```python
from build123d import *

# Parameters (mm, degrees)
BOSS_EXTRUDE1_DEPTH    = 3.81
F_10_CLEARANCE_HOLE1_D = 5.1054
F_6_32_TAPPED_HOLE1_D  = 2.7051
SKETCH4_R              = 3.175
CUT_EXTRUDE1_DEPTH     = 33.948179104


with BuildPart() as part:
    # Sketch1 → Boss-Extrude1 (new body)
    with BuildSketch(Plane(origin=(0, 0, 0), x_dir=(0, 0, -1), z_dir=(1, 0, 0))):
        with BuildLine():
            ThreePointArc((-25.906015625, 4.73554162), (-30.1625, 0), (-25.906015625, -4.73554162))
            ThreePointArc((-25.906015625, -4.73554162), (-15.759385528, -6.884569442), (-6.260703125, -11.049597114))
            ThreePointArc((-6.260703125, -11.049597114), (0, -12.7), (6.260703125, -11.049597114))
            ThreePointArc((6.260703125, -11.049597114), (15.759385528, -6.884569442), (25.906015625, -4.73554162))
            ThreePointArc((25.906015625, -4.73554162), (30.1625, 0), (25.906015625, 4.73554162))
            ThreePointArc((25.906015625, 4.73554162), (15.759385528, 6.884569442), (6.260703125, 11.049597114))
            ThreePointArc((6.260703125, 11.049597114), (0, 12.7), (-6.260703125, 11.049597114))
            ThreePointArc((-6.260703125, 11.049597114), (-15.759385528, 6.884569442), (-25.906015625, 4.73554162))
        make_face()
    extrude(amount=-BOSS_EXTRUDE1_DEPTH)

    # #10 Clearance Hole1 (through all)
    with Locations(Plane.ZY.offset(3.81)):
        with Locations((-25.4, 0), (25.4, 0)):
            Hole(F_10_CLEARANCE_HOLE1_D / 2)

    # #6-32 Tapped Hole1 (through all)
    with Locations(Plane.ZY.offset(3.81)):
        with Locations((0, -5.715)):
            Hole(F_6_32_TAPPED_HOLE1_D / 2)

    # Sketch4 → Cut-Extrude1 (cut, through all)
    with BuildSketch(Plane.ZY.offset(3.81)):
        Circle(SKETCH4_R)
    extrude(amount=-CUT_EXTRUDE1_DEPTH, mode=Mode.SUBTRACT)


solid = part.part
```
For this review, take the finished solid that the model builds, in its own axes (mm). Coordinates: 2 decimals unless noted, no trailing zeros. Write each loop counter-clockwise with the first axis right and the second up, starting at its lowest first coordinate (ties: lowest second). Pieces come first, ordered by that corner, then holes. Notation, with made-up numbers: (4.5, -13.75) -> (15.5, -13.75) arc R31 ccw to (15.5, 19.25) -> close; hole circle Ø11 at (-22.75, -39.75). An arc over 180 degrees is marked (long way). Put each result on its own line as item: value.
Q1. Take a section at D-D, the plane y = 9.25. State the section outline as (x, z) points.
From the geometry:
outline: (-3.81, -9.74) -> (0, -9.74) -> (0, 9.74) -> (-3.81, 9.74) -> close
Q2. Take a section at A-A, the plane z = 0. State the section outline as (x, y) points (3 decimals), then the cut area to 3 significant figures.
From the geometry:
outline: (-3.81, -12.7) -> (0, -12.7) -> (0, -7.068) -> (-3.81, -7.068) -> close; (-3.81, -4.362) -> (0, -4.362) -> (0, -3.175) -> (-3.81, -3.175) -> close; (-3.81, 3.175) -> (0, 3.175) -> (0, 12.7) -> (-3.81, 12.7) -> close
area: 62.3 mm2
Q3. Wall thickness on L1, parallel to Y at x = -1.8, z = 0 (3 decimals); L2, parallel to Z at x = -0.85, y = -0.75; L3, parallel to Y at x = -2.75, z = 25.5: over which ranges is each line inside the solid? List them lowest first.
From the geometry:
L1: y = -12.7 to -7.068, -4.362 to -3.175, 3.175 to 12.7
L2: z = -30.1 to -27.84, -22.96 to -3.09, 3.09 to 22.96, 27.84 to 30.1
L3: y = -4.78 to -2.55, 2.55 to 4.78
Q4. Take a section at C-C, the plane z = -24. State the section outline as (x, y) points.
From the geometry:
outline: (-3.81, -4.98) -> (0, -4.98) -> (0, -2.13) -> (-3.81, -2.13) -> close; (-3.81, 2.13) -> (0, 2.13) -> (0, 4.98) -> (-3.81, 4.98) -> close
Q5. Take a section at B-B, the plane y = 0. State the section outline as (x, z) points (1 decimal), then the cut area to 3 significant figures.
From the geometry:
outline: (-3.8, -30.2) -> (0, -30.2) -> (0, -28) -> (-3.8, -28) -> close; (-3.8, -22.8) -> (0, -22.8) -> (0, -3.2) -> (-3.8, -3.2) -> close; (-3.8, 3.2) -> (0, 3.2) -> (0, 22.8) -> (-3.8, 22.8) -> close; (-3.8, 28) -> (0, 28) -> (0, 30.2) -> (-3.8, 30.2) -> close
area: 167 mm2
Q6. The part is to be moulded in two halves that separate along Z. For faces 1 (the cylindrical face through (-1.88, -6.93, -15.62)), 2 (the cylindrical face through (-1.9, -12.7, 0.1)), 3 (the cylindrical face through (-1.88, -6.84, 15.9)), 4 (the cylindrical face through (-1.93, -3.1, -0.69)), say which applies: +Z half, -Z half, draft (parallel to the pull), parting line (faces both ways), or undercut.
From the geometry:
face 1: -Z half
face 2: parting line
face 3: +Z half
face 4: undercut
